Model file for the job. Use its own axes, mm. Face numbers are marked on the shaded views. A direction names the side the tool comes from. Give positions to 0.01 mm unless a question says otherwise; leave off trailing zeros. Write each loop counter-clockwise with the first axis right and the second up, starting at its lowest first coordinate (ties: lowest second). Pieces come first, ordered by that corner, then holes. Notation, with made-up numbers: (6.5, 23) - (56.5, 23) arc R31 ccw to (56.5, 57) - close; hole circle Ø6 at (88, 56). An arc over 180 degrees is marked (long way). Use CSV: the item, a comma, the result in double quotes.
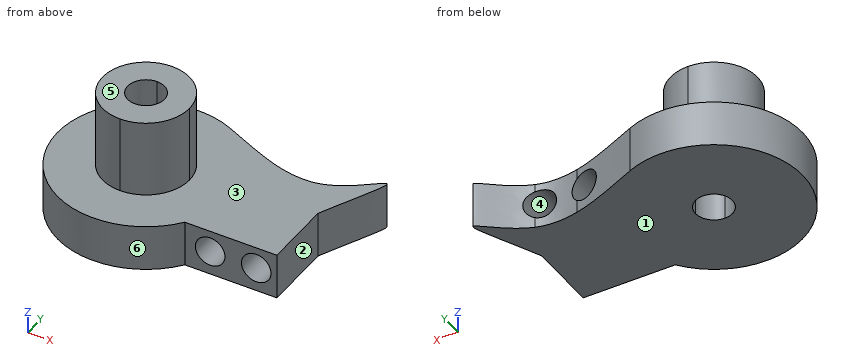
from build123d import *

# Parameters (mm, degrees)
F1_DEPTH = 25
F2_DEPTH = 67
F3_R     = 8.0170654264
F4_DEPTH = 77.2782947511


with BuildPart() as f1:
    # F0 (on Top) → F1 (new body)
    with BuildSketch(Plane.XY):
        with BuildLine():
            Line((-44.1382192087, 23.6139522209), (-44.1382192087, 29.1501541541))
            Line((-44.1382192087, 29.1501541541), (-5.8434393396, 29.1501541541))
            ThreePointArc((-5.8434393396, 29.1501541541), (-14.3812854567, 37.8252104568), (-24.8224606144, 44.080870254))
            ThreePointArc((-24.8224606144, 44.080870254), (-90.7261926511, -12.074037558), (-5.8434393396, -29.1501541541))
            Line((-5.8434393396, -29.1501541541), (-44.1382192087, -29.1501541541))
            Line((-44.1382192087, -29.1501541541), (-44.1382192087, -23.6139522209))
            ThreePointArc((-44.1382192087, -23.6139522209), (-67.7521714295, 0), (-44.1382192087, 23.6139522209))
        make_face()
        with BuildLine():
            Line((12.8327377156, 29.1501541541), (-5.8434393396, 29.1501541541))
            ThreePointArc((-5.8434393396, 29.1501541541), (1.4646310503, 15.3818627182), (3.9889212884, 0))
            ThreePointArc((3.9889212884, 0), (1.4646310503, -15.3818627182), (-5.8434393396, -29.1501541541))
            Line((-5.8434393396, -29.1501541541), (44.1382192087, -29.1501541541))
            Line((44.1382192087, -29.1501541541), (44.1382192087, 8.3397841081))
            Line((44.1382192087, 8.3397841081), (44.1382192087, 29.1501541541))
            Line((44.1382192087, 29.1501541541), (35.5350334868, 29.1501541541))
            add(Edge.make_bspline(
                [(12.8327377156, 29.1501541541), (20.8092349471, 27.208546417), (28.4195513087, 26.8060990258), (35.5350334868, 29.1501541541)],
                knots=[0.2413128636, 0.2413128636, 0.2413128636, 0.2413128636, 0.4033216227, 0.4033216227, 0.4033216227, 0.4033216227], degree=3))
        make_face()
        with BuildLine():
            add(Edge.make_bspline(
                [(35.5350334868, 29.1501541541), (47.6218028789, 33.1319017108), (70.7323680982, 58.9476120465), (52.2453960839, 26.1592553027), (44.1382192087, 8.3397841081)],
                knots=[0.4033216227, 0.4033216227, 0.4033216227, 0.4033216227, 0.6785190669, 1, 1, 1, 1], degree=3))
            Line((35.5350334868, 29.1501541541), (44.1382192087, 29.1501541541))
            Line((44.1382192087, 29.1501541541), (44.1382192087, 8.3397841081))
        make_face()
        with BuildLine():
            ThreePointArc((-24.8224606144, 44.080870254), (-14.3812854567, 37.8252104568), (-5.8434393396, 29.1501541541))
            Line((-5.8434393396, 29.1501541541), (12.8327377156, 29.1501541541))
            add(Edge.make_bspline(
                [(-24.8224606144, 44.080870254), (-11.7417461231, 38.3490432302), (0.9517048626, 32.0421886703), (12.8327377156, 29.1501541541)],
                knots=[0, 0, 0, 0, 0.2413128636, 0.2413128636, 0.2413128636, 0.2413128636], degree=3))
        make_face()
        with BuildLine():
            Line((-5.8434393396, 29.1501541541), (-44.1382192087, 29.1501541541))
            Line((-44.1382192087, 29.1501541541), (-44.1382192087, 23.6139522209))
            ThreePointArc((-44.1382192087, 23.6139522209), (-27.4406334627, 16.697585746), (-20.5242669878, 0))
            ThreePointArc((-20.5242669878, 0), (-27.4406334627, -16.697585746), (-44.1382192087, -23.6139522209))
            Line((-44.1382192087, -23.6139522209), (-44.1382192087, -29.1501541541))
            Line((-44.1382192087, -29.1501541541), (-5.8434393396, -29.1501541541))
            ThreePointArc((-5.8434393396, -29.1501541541), (1.4646310503, -15.3818627182), (3.9889212884, 0))
            ThreePointArc((3.9889212884, 0), (1.4646310503, 15.3818627182), (-5.8434393396, 29.1501541541))
        make_face()
    extrude(amount=F1_DEPTH)

    # F0 (on Top) → F2 (join)
    with BuildSketch(Plane.XY):
        with BuildLine():
            Line((-44.1382192087, 10), (-44.1382192087, 23.6139522209))
            ThreePointArc((-44.1382192087, 23.6139522209), (-67.7521714295, 0), (-44.1382192087, -23.6139522209))
            Line((-44.1382192087, -23.6139522209), (-44.1382192087, -10))
            ThreePointArc((-44.1382192087, -10), (-54.1382192087, 0), (-44.1382192087, 10))
        make_face()
        with BuildLine():
            ThreePointArc((-20.5242669878, 0), (-27.4406334627, 16.697585746), (-44.1382192087, 23.6139522209))
            Line((-44.1382192087, 23.6139522209), (-44.1382192087, 10))
            ThreePointArc((-44.1382192087, 10), (-37.0671513968, 7.0710678119), (-34.1382192087, 0))
            ThreePointArc((-34.1382192087, 0), (-37.0671513968, -7.0710678119), (-44.1382192087, -10))
            Line((-44.1382192087, -10), (-44.1382192087, -23.6139522209))
            ThreePointArc((-44.1382192087, -23.6139522209), (-27.4406334627, -16.697585746), (-20.5242669878, 0))
        make_face()
    extrude(amount=F2_DEPTH)

    # F3 (on face) → F4 (cut, through all)
    with BuildSketch(Plane.XZ.offset(29.1501541541)):
        with Locations((7.9276636243, 13.1636038423)):
            Circle(F3_R)
        with Locations((32.9276636243, 13.1636038423)):
            Circle(F3_R)
    extrude(amount=-F4_DEPTH, mode=Mode.SUBTRACT)


solid = f1.part
(1) Pull direction Z, two halves, no side cores. Call the marked faces 4, 5 and 6: released by +Z, released by -Z, zero draft, split by the parting line, or undercut.
Checked values:
face 4,"undercut"
face 5,"released by +Z"
face 6,"zero draft"
(2) Flat gauge pins, fed straight in: P1, Ø3, axis at x = -28.5, z = 60.5, coming from the -Y side; P2, Ø4, axis at x = 8, y = 16, coming from the +Z side; P3, Ø4, axis at y = -6, z = 12, coming from the +X side. Where does each tip first touch, or does it go through?
Checked values:
P1,"stops at y = -18.91"
P2,"stops at z = 25"
P3,"stops at x = 44.14"
(3) 3-axis set-ups, long thin cutter, end or side, ignore diameter. For the marked faces 1, 2 and 3: which of +Z, -Z, +X, -X, +Y, -Y reach the whole face in a straight line?
Checked values:
face 1,"-Z, +X, -X, +Y, -Y"
face 2,"+Z, -Z, +X, -Y"
face 3,"+Z"
(4) Saw through at D-D, the plane x = -80. List the corners of the cut face in (y, z).
Checked values:
outline,"(-32.1, 0) - (32.1, 0) - (32.1, 25) - (-32.1, 25) - close"
(5) Saw through at C-C, the plane y = -41.5. List the corners of the cut face in (x, z).
Checked values:
outline,"(-68.51, 0) - (-19.77, 0) - (-19.77, 25) - (-68.51, 25) - close"
(6) Saw through at A-A, the plane x = -47. List the corners of the cut face in (y, z).
Checked values:
outline,"(-48.04, 0) - (-9.58, 0) - (-9.58, 67) - (-23.44, 67) - (-23.44, 25) - (-48.04, 25) - close; (9.58, 0) - (48.04, 0) - (48.04, 25) - (23.44, 25) - (23.44, 67) - (9.58, 67) - close"
(7) Wall check: probe 1 along X at (y, z) = (-1, 20); probe 2 along X at (y, z) = (-2.5, 7.5); probe 3 along X at (y, z) = (13, 7). Give the ranges that are in metal, low to high. Write a range as [from, to].
Checked values:
probe 1,"x = [-92.25, -54.09], [-34.19, 3.74], [12.12, 28.74], [37.12, 44.14]"
probe 2,"x = [-92.2, -53.82], [-34.46, 2.25], [13.6, 27.25], [38.6, 44.14]"
probe 3,"x = [-90.48, 2.8], [13.05, 27.8], [38.05, 46.3]"
(8) Saw through at B-B, the plane y = -20. List the corners of the cut face in (x, z), then the cut area to 3 significant figures.
Checked values:
outline,"(-87.91, 0) - (44.14, 0) - (44.14, 25) - (-31.58, 25) - (-31.58, 67) - (-56.69, 67) - (-56.69, 25) - (-87.91, 25) - close; hole circle Ø16.03 at (7.93, 13.16); hole circle Ø16.03 at (32.93, 13.16)"
area,"3,950 mm^2"
